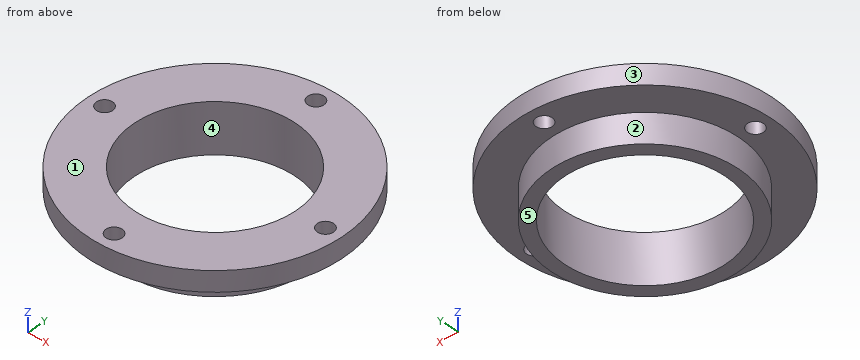
Solid Edge part; units mm, degrees
sketch "Sketch1" plane through (0, 0, 0) normal (0, -1, 0) x (1, 0, 0)
  line L0 (19, 17) -> (14, 17)
  line L1 (14, 17) -> (14, 12.6275)
  line L2 (14, 12.6275) -> (12, 12.6275)
  line L3 (12, 20) -> (12, 12.6275)
  line L4 (12, 20) -> (19, 20)
  line L5 (19, 20) -> (19, 17)
revolve "RevolvedProtrusion1" add sketch "Sketch1" angle 360 about axis through (0, 0, 11.8307) along (0, 0, 1)
hole "Hole1" at (-16.52, 0, 20) direction (0, 0, -1) diameter 2.4 end through all
pattern_circular "Pattern1" count 4 over 360 about axis through (0, 0, 20) along (0, 0, -1) of "Hole1"
cosmetic_thread "Thread1"
Here's how the part is built. I have some questions about the finished solid (model axes, mm). Face numbers are marked on the shaded views. A direction names the side the tool comes from. Give positions to 0.01 mm unless a question says otherwise; leave off trailing zeros. Order: outer loops, then holes, each group sorted by start corner. A loop starts at its lowest first (then second) coordinate and runs counter-clockwise, first axis right, second up. Notation, with made-up numbers: (52, 24) -> (77, 24) arc R11 cw to (77, 35) -> close; hole circle Ø1 at (65, 66.5). An arc over 180 degrees is marked (long way). Use a Markdown table: item, result. Add a question column.
Item 1: Imagine slicing it at C-C on x = 7.5. Please give me the cut outline in (y, z), plus the area to 3 significant figures.
Item 2: Will these pins go through, and if not, where does the flat tip stop? pin 1 (11.5 mm diameter, centred on x = 4.5, y = 7.5, fed in from -Z); pin 2 (2 mm diameter, centred on x = 0, y = -16.52, fed in from -Z); pin 3 (1.5 mm diameter, centred on x = -2.5, z = 13.5, fed in from +Y).
Item 3: Imagine slicing it at A-A on x = 0. Please give me the cut outline in (y, z), plus the area to 3 significant figures.
Item 4: Imagine slicing it at D-D on z = 17.75. Please give me the cut outline in (x, y), plus the area to 3 significant figures.
Item 5: If we mould it in two halves opening along X, with no side actions, what happens to the marked faces 3, 4 and 5? For each: pulls with the +X half, pulls with the -X half, needs draft (parallel to the pull), parting line crosses it, or undercut.
Item 6: I need wall thicknesses on line 1 (Y direction, x = 0, z = 17.8); line 2 (Y direction, x = 7.5, z = 15.25); line 3 (Y direction, x = 16.52, z = 19.4). Which ranges of each line are inside material? Lowest first, please.
Item 7: For the marked faces 1 and 2, which set-ups out of +Z, -Z, +X, -X, +Y, -Y let a thin tool reach every point of the face, with its end or its side?
Data:
| question | item | result |
|---|---|---|
| 1 | outline | (-17.46, 17) -> (-11.82, 17) -> (-11.82, 12.63) -> (-9.37, 12.63) -> (-9.37, 20) -> (-17.46, 20) -> close; (9.37, 12.63) -> (11.82, 12.63) -> (11.82, 17) -> (17.46, 17) -> (17.46, 20) -> (9.37, 20) -> close |
| 1 | area | 70.0 mm² |
| 2 | pin 1 | stops at z = 12.63 |
| 2 | pin 2 | passes through |
| 2 | pin 3 | stops at y = 13.89 |
| 3 | outline | (-19, 17) -> (-17.72, 17) -> (-17.72, 20) -> (-19, 20) -> close; (-15.32, 17) -> (-14, 17) -> (-14, 12.63) -> (-12, 12.63) -> (-12, 20) -> (-15.32, 20) -> close; (12, 12.63) -> (14, 12.63) -> (14, 17) -> (15.32, 17) -> (15.32, 20) -> (12, 20) -> close; (17.72, 17) -> (19, 17) -> (19, 20) -> (17.72, 20) -> close |
| 3 | area | 45.1 mm² |
| 4 | outline | circle Ø38 at (0, 0); hole circle Ø2.4 at (-16.52, 0); hole circle Ø24 at (0, 0); hole circle Ø2.4 at (0, -16.52); hole circle Ø2.4 at (0, 16.52); hole circle Ø2.4 at (16.52, 0) |
| 4 | area | 664 mm² |
| 5 | face 3 | parting line crosses it |
| 5 | face 4 | undercut |
| 5 | face 5 | needs draft |
| 6 | line 1 | y = -19 to -17.72, -15.32 to -12, 12 to 15.32, 17.72 to 19 |
| 6 | line 2 | y = -11.82 to -9.37, 9.37 to 11.82 |
| 6 | line 3 | y = -9.39 to -1.2, 1.2 to 9.39 |
| 7 | face 1 | +Z, +X, -X, +Y, -Y |
| 7 | face 2 | -Z |
